```python
from build123d import *

# Parameters (mm, degrees)
BOSS_EXTRUDE1_DEPTH = 42
SKETCH2_W           = 25
SKETCH2_H           = 71
CUT_EXTRUDE1_DEPTH  = 108.391806019
CUT_EXTRUDE2_REACH  = 101.363
SKETCH4_R           = 1.7
SKETCH7_R           = 2.6
CUT_EXTRUDE3_DEPTH  = 10
FILLET1_R           = 3
FILLET2_R           = 3
SKETCH8_W           = 39
SKETCH8_H           = 36
CUT_EXTRUDE4_DEPTH  = 14


with BuildPart() as part:
    # Sketch1 → Boss-Extrude1 (new body)
    with BuildSketch(Plane.XY):
        Polygon((10, 17), (45, 17), (45, 0), (0, 0), (0, 88), (33, 88), (33, 78), (39, 78), (39, 88), (44, 88), (44, 73), (10, 73), align=None)
    extrude(amount=BOSS_EXTRUDE1_DEPTH)

    # Sketch2 → Cut-Extrude1 (cut, through all)
    with BuildSketch(Plane.ZY):
        with Locations((21, 52.5)):
            Rectangle(SKETCH2_W, SKETCH2_H)
    extrude(amount=-CUT_EXTRUDE1_DEPTH, mode=Mode.SUBTRACT)

    # Sketch4 → Cut-Extrude2 (cut, up to next)
    with BuildSketch(Plane(origin=(0, 78, 0), x_dir=(1, 0, 0), z_dir=(0, 1, 0)), mode=Mode.PRIVATE) as cut_extrude2_sk1:
        with Locations(Location((36, -37.75, 0), (0, 0, 270))):
            Circle(SKETCH4_R)
    cut_extrude2_tool1 = extrude(cut_extrude2_sk1.sketch, amount=-CUT_EXTRUDE2_REACH, mode=Mode.PRIVATE) & part.part
    # Sketch4 → Cut-Extrude2 (cut, up to next)
    with BuildSketch(Plane(origin=(0, 78, 0), x_dir=(1, 0, 0), z_dir=(0, 1, 0)), mode=Mode.PRIVATE) as cut_extrude2_sk2:
        with Locations(Location((36, -4.25, 0), (0, 0, 270))):
            Circle(SKETCH4_R)
    cut_extrude2_tool2 = extrude(cut_extrude2_sk2.sketch, amount=-CUT_EXTRUDE2_REACH, mode=Mode.PRIVATE) & part.part
    add(cut_extrude2_tool1.solids().sort_by_distance((36, 78, 37.75))[0], mode=Mode.SUBTRACT)
    add(cut_extrude2_tool2.solids().sort_by_distance((36, 78, 4.25))[0], mode=Mode.SUBTRACT)

    # Sketch7 → Cut-Extrude3 (cut)
    with BuildSketch(Plane(origin=(45, 0, 0), x_dir=(0, 0, -1), z_dir=(1, 0, 0))):
        with Locations((-32.5, 8.5)):
            Circle(SKETCH7_R)
    extrude(amount=-CUT_EXTRUDE3_DEPTH, mode=Mode.SUBTRACT)

    # Fillet1
    fillet1_edges = [part.edges().sort_by_distance(p)[0] for p in [
        (10, 17, 37.75),
        (10, 17, 4.25),
        (5, 17, 33.5),
        (5, 17, 8.5),
    ]]
    fillet(fillet1_edges, radius=FILLET1_R)

    # Fillet2
    fillet2_edges = [part.edges().sort_by_distance(p)[0] for p in [
        (44, 73, 37.75),
        (10, 73, 37.75),
        (44, 73, 4.25),
        (10, 73, 4.25),
    ]]
    fillet(fillet2_edges, radius=FILLET2_R)

    # Sketch8 → Cut-Extrude4 (cut)
    with BuildSketch(Plane.XZ):
        with Locations((22.5, 21)):
            Rectangle(SKETCH8_W, SKETCH8_H)
    extrude(amount=-CUT_EXTRUDE4_DEPTH, mode=Mode.SUBTRACT)


solid = part.part
```
Source: CAD feature listing. Evaluate the final solid. Frame: model axes, mm. A direction names the side the tool comes from. Give positions to 0.01 mm unless a question says otherwise; leave off trailing zeros. Loops run counter-clockwise (first coordinate to the right, second up) from the corner with the lowest first, then second, coordinate; pieces in that order, holes last. Notation, with made-up numbers: (70, 36) - (117, 36) arc R17 cw to (117, 67) - close; hole circle Ø11 at (67, 15.5). An arc over 180 degrees is marked (long way). Use CSV: the item, a comma, the result in double quotes. Start each with the question number.
1. Section A-A (x = 36). Output: boundary loops of the cut face in (y, z), then the cut area to 3 significant figures.
2. Draft query along X for faces 1 (the flat face through (22, 14, 21)), 2 (the cylindrical face through (10.9, 17.86, 37.61)), 3 (the flat face through (7, 61, 8.5)), 4 (the flat face through (39, 83, 4)). Return one class per face: +X half, -X half, draft (parallel to the pull), parting line (faces both ways), or undercut.
3. Section B-B (z = 4.25). Output: boundary loops of the cut face in (x, y), then the cut area to 3 significant figures.
4. Reachability of faces 5 (the flat face through (33, 83, 38)), 6 (the cylindrical face through (5.15, 17.86, 9.4)), 7 (the flat face through (22, 7, 39)) from +Z, -Z, +X, -X, +Y, -Y: full face, straight path, thin tool, end or side. Return the list, or none.
5. Section C-C (y = 61). Output: boundary loops of the cut face in (x, z).
6. Section D-D (x = 19). Output: boundary loops of the cut face in (y, z), then the cut area to 3 significant figures.
7. Pin query (flat end, axial travel): pin 1 (2.5 mm diameter, centred on y = 43, z = 36.5, fed in from +X); pin 2 (12.5 mm diameter, centred on x = 15, z = 21.5, fed in from +Y); pin 3 (2 mm diameter, centred on x = 24.5, z = 12.5, fed in from -Y); pin 4 (4 mm diameter, centred on x = 28, z = 37.5, fed in from -Y). Return the tip coordinate at first contact, or that it passes through.
8. Ray query, L1, parallel to X at y = 76, z = 4; L2, parallel to Z at x = 19, y = 77.5; L3, parallel to Y at x = 32, z = 7. Return the intervals inside material, ascending.
Response:
1,outline,"(0, 0) - (17, 0) - (17, 42) - (0, 42) - (0, 39) - (14, 39) - (14, 3) - (0, 3) - close; (73, 0) - (78, 0) - (78, 2.55) - (73, 2.55) - close; (73, 5.95) - (78, 5.95) - (78, 8.5) - (73, 8.5) - close; (73, 33.5) - (78, 33.5) - (78, 36.05) - (73, 36.05) - close; (73, 39.45) - (78, 39.45) - (78, 42) - (73, 42) - close"
1,area,"261 mm²"
2,face 1,"undercut"
2,face 2,"+X half"
2,face 3,"draft"
2,face 4,"undercut"
3,outline,"(0, 0) - (3, 0) - (3, 14) - (42, 14) - (42, 0) - (45, 0) - (45, 17) - (13, 17) arc R3 cw to (10, 20) - (10, 70) arc R3 cw to (13, 73) - (34.3, 73) - (34.3, 78) - (33, 78) - (33, 88) - (0, 88) - close; (37.7, 73) - (41, 73) arc R3 ccw to (44, 76) - (44, 88) - (39, 88) - (39, 78) - (37.7, 78) - close"
3,area,"1,360 mm²"
4,face 5,"+Z, -Z, +Y"
4,face 6,"+X, -X, +Y"
4,face 7,"-Y"
5,outline,"(0, 0) - (10, 0) - (10, 8.5) - (0, 8.5) - close; (0, 33.5) - (10, 33.5) - (10, 42) - (0, 42) - close"
6,outline,"(0, 0) - (17, 0) - (17, 42) - (0, 42) - (0, 39) - (14, 39) - (14, 3) - (0, 3) - close; (73, 0) - (88, 0) - (88, 8.5) - (73, 8.5) - close; (73, 33.5) - (88, 33.5) - (88, 42) - (73, 42) - close"
6,area,"465 mm²"
7,pin 1,"x = 10"
7,pin 2,"y = 17"
7,pin 3,"y = 14"
7,pin 4,"y = 0"
8,L1,"0 to 34.32, 37.68 to 44"
8,L2,"0 to 8.5, 33.5 to 42"
8,L3,"14 to 17, 73 to 88"
